```python
from build123d import *

# Parameters (mm, degrees)
SKETCH_1_W          = 1596
SKETCH_1_H          = 590
EXTRUDE_1_DEPTH     = 2
EXTRUDE_2_DEPTH     = 90
EXTRUDE_5_DEPTH     = 96
CUT_EXTRUDE_1_DEPTH = 94


with BuildPart() as part:
    # 草图1 → 凸台-拉伸1 (new body)
    with BuildSketch(Plane.XY):
        Rectangle(SKETCH_1_W, SKETCH_1_H)
    extrude(amount=EXTRUDE_1_DEPTH)

    # 草图2 → 凸台-拉伸2 (add)
    with BuildSketch(Plane.XY.offset(2)):
        Polygon((-798, -293), (796, -293), (798, -293), (798, -295), (-798, -295), align=None)
        Polygon((796, 293), (798, 293), (798, 295), (-798, 295), (-798, 293), align=None)
    extrude(amount=EXTRUDE_2_DEPTH)

    # 草图5 → 凸台-拉伸5 (add)
    with BuildSketch(Plane(origin=(0, 0, 0), x_dir=(-1, 0, 0), z_dir=(0, 0, -1))):
        with BuildLine():
            Line((798, 295), (798, -295))
            ThreePointArc((798, -295), (1198.010532784, 20.610905531), (1183.918362251, 529.943881843))
            ThreePointArc((1183.918362251, 529.943881843), (1078.504933407, 588.278536691), (981.833490458, 516.378918785))
            ThreePointArc((981.833490458, 516.378918785), (908.585128619, 390.187197034), (798, 295))
        make_face()
    extrude(amount=-EXTRUDE_5_DEPTH)

    # 草图6 → 切除-拉伸1 (cut)
    with BuildSketch(Plane.XY.offset(96)):
        with BuildLine():
            Line((-797.998398705, 292.662145907), (-797.597225993, -293.040976493))
            ThreePointArc((-797.597225993, -293.040976493), (-1196.198962172, 21.458379377), (-1182.156422838, 528.997536503))
            ThreePointArc((-1182.156422838, 528.997536503), (-1078.638882134, 586.283027298), (-983.706100418, 515.67654286))
            ThreePointArc((-983.706100418, 515.67654286), (-910.123787085, 388.909492011), (-799.034482428, 293.288320677))
            Line((-799.034482428, 293.288320677), (-797.998398705, 292.662145907))
        make_face()
    extrude(amount=-CUT_EXTRUDE_1_DEPTH, mode=Mode.SUBTRACT)


solid = part.part
```
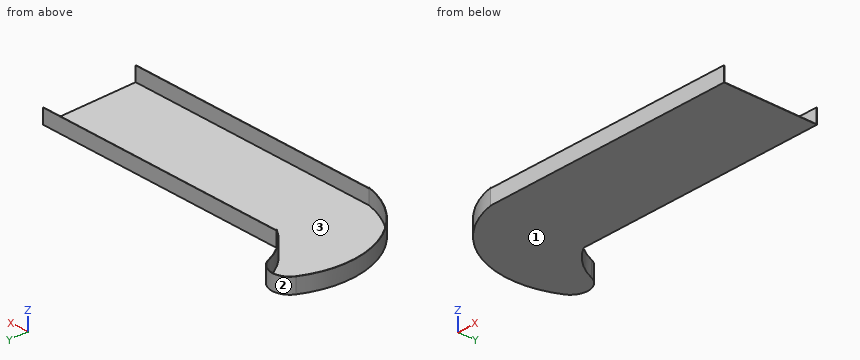
Work out the finished part from the listing and answer in its coordinate system (mm). Face numbers are marked on the shaded views. Give positions to 0.01 mm unless a question says otherwise; leave off trailing zeros. Loops run counter-clockwise (first coordinate to the right, second up) from the corner with the lowest first, then second, coordinate; pieces in that order, holes last. Notation, with made-up numbers: (15.25, 82) -> (52.25, 82) arc R4 cw to (52.25, 86) -> close; hole circle Ø9 at (54.25, 34). An arc over 180 degrees is marked (long way). Put each result on its own line as item: value. Start each with the question number.
Item 1: The part is cut by section B-B (x = 204). Give the vertices of the cut face in (y, z), then the cut area to 3 significant figures.
Item 2: The part is cut by section A-A (z = 73). Give the vertices of the cut face in (x, y).
Item 3: Each of these flat-tipped pins is pushed along its axis until it touches: P1, Ø12, axis at y = 228, z = 29.5, coming from the +X side; P2, Ø6, axis at x = 16.5, z = 85.5, coming from the +Y side; P3, Ø1.6, axis at x = -148.5, y = -293.5, coming from the +Z side. Where does it stop, or does it pass through?
Item 4: The part is cut by section D-D (y = 42). Give the vertices of the cut face in (x, z).
Item 5: The mould has two halves that part along Y. Classify the marked faces 1, 2 and 3: released by +Y, released by -Y, zero draft, split by the parting line, or undercut.
Item 6: Find the intervals of material crossed by L1, parallel to Y at x = -742, z = 57.5; L2, parallel to Z at x = -994, y = 526; L3, parallel to Y at x = -1134.5, z = 20, in increasing order. Write a range as [from, to].
Item 7: The part is cut by section C-C (y = 335). Give the vertices of the cut face in (x, z), then the cut area to 3 significant figures.
Answers below:
1. outline: (-295, 0) -> (295, 0) -> (295, 92) -> (293, 92) -> (293, 2) -> (-293, 2) -> (-293, 92) -> (-295, 92) -> close
1. area: 1,540 mm2
2. outline: (-1183.92, 529.94) arc R567.88 ccw to (-798, -295) -> (798, -295) -> (798, -293) -> (-797.6, -293) -> (-797.6, -293.04) arc R565.88 cw to (-797.8, -293) -> (-798, -293) -> (-798, -292.96) arc R565.88 cw to (-1182.16, 529) arc R109.2 cw to (-983.71, 515.68) arc R440.68 ccw to (-799.03, 293.29) -> (-798, 292.66) -> (-798, 293) -> (798, 293) -> (798, 295) -> (-798, 295) arc R438.68 cw to (-981.83, 516.38) arc R111.2 ccw to start
3. P1: x = -1248.15
3. P2: y = 295
3. P3: z = 92
4. outline: (-1207.48, 0) -> (798, 0) -> (798, 2) -> (-1205.32, 2) -> (-1205.32, 96) -> (-1207.48, 96) -> close
5. face 1: zero draft
5. face 2: released by +Y
5. face 3: undercut
6. L1: [-295, -293], [293, 295]
6. L2: [0, 2]
6. L3: [-84.02, -80.72], [575.14, 577.37]
7. outline: (-1246.7, 0) -> (-853.8, 0) -> (-853.8, 96) -> (-856.89, 96) -> (-856.89, 2) -> (-1244.69, 2) -> (-1244.69, 96) -> (-1246.7, 96) -> close
7. area: 1,270 mm2
